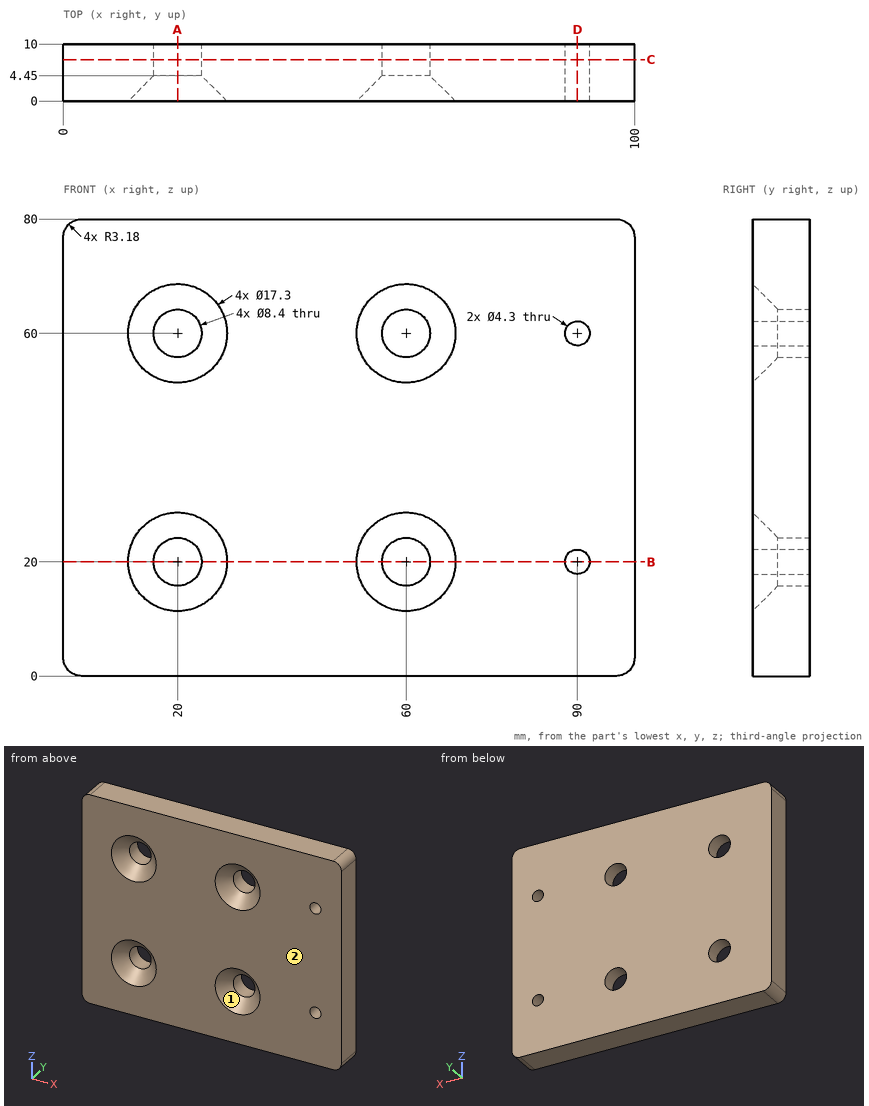
Drawing for the job (mm, zero at the part's lowest x, y, z). Round coordinates to 2 decimals unless told otherwise and drop trailing zeros. Order: outer loops, then holes, each group sorted by start corner. A loop starts at its lowest first (then second) coordinate and runs counter-clockwise, first axis right, second up.
Item 1: Probe line 1 along X through (y, z) = (7.3, 20); line 2 along Z through (x, y) = (60, 7.9); line 3 along Z through (x, y) = (90, 7). List the from-to ranges inside material, lowest first.
Item 2: Saw through at A-A on x = 20. Write the cut outline in (y, z), then the cut area to 3 significant figures.
Item 3: Saw through at D-D on x = 90. Write the cut outline in (y, z), then the cut area to 3 significant figures.
Item 4: Saw through at B-B on z = 20. Write the cut outline in (x, y), then the cut area to 3 significant figures.
Item 5: Saw through at C-C on y = 7.25. Write the cut outline in (x, z).
Item 6: Mould opens along Z. For the marked faces 1 and 2 say: pulls with the +Z half, pulls with the -Z half, needs draft (parallel to the pull), parting line crosses it, or undercut.
Reported:
1. line 1: x = 0 to 15.8, 24.2 to 55.8, 64.2 to 87.85, 92.15 to 100
1. line 2: z = 0 to 15.8, 24.2 to 55.8, 64.2 to 80
1. line 3: z = 0 to 17.85, 22.15 to 57.85, 62.15 to 80
2. outline: (0, 0) - (10, 0) - (10, 15.8) - (4.45, 15.8) - (0, 11.35) - close; (0, 28.65) - (4.45, 24.2) - (10, 24.2) - (10, 55.8) - (4.45, 55.8) - (0, 51.35) - close; (0, 68.65) - (4.45, 64.2) - (10, 64.2) - (10, 80) - (0, 80) - close
2. area: 592 mm2
3. outline: (0, 0) - (10, 0) - (10, 17.85) - (0, 17.85) - close; (0, 22.15) - (10, 22.15) - (10, 57.85) - (0, 57.85) - close; (0, 62.15) - (10, 62.15) - (10, 80) - (0, 80) - close
3. area: 714 mm2
4. outline: (0, 0) - (11.35, 0) - (15.8, 4.45) - (15.8, 10) - (0, 10) - close; (24.2, 4.45) - (28.65, 0) - (51.35, 0) - (55.8, 4.45) - (55.8, 10) - (24.2, 10) - close; (64.2, 4.45) - (68.65, 0) - (87.85, 0) - (87.85, 10) - (64.2, 10) - close; (92.15, 0) - (100, 0) - (100, 10) - (92.15, 10) - close
4. area: 749 mm2
5. outline: (0, 3.18) arc R3.18 ccw to (3.18, 0) - (96.82, 0) arc R3.18 ccw to (100, 3.18) - (100, 76.82) arc R3.18 ccw to (96.82, 80) - (3.18, 80) arc R3.18 ccw to (0, 76.82) - close; hole circle Ø8.4 at (20, 20); hole circle Ø8.4 at (20, 60); hole circle Ø8.4 at (60, 20); hole circle Ø8.4 at (60, 60); hole circle Ø4.3 at (90, 20); hole circle Ø4.3 at (90, 60)
6. face 1: undercut
6. face 2: needs draft
